```python
from build123d import *

# Parameters (mm, degrees)
SKETCH1_R           = 2.1
BOSS_EXTRUDE1_DEPTH = 2.38
BOSS_EXTRUDE2_START = 2.38
SKETCH1_3_W         = 40.25
SKETCH1_3_H         = 19.88
SKETCH1_3_W_2       = 6.925
SKETCH1_3_H_2       = 0.92
BOSS_EXTRUDE2_DEPTH = 5.72
BOSS_EXTRUDE3_START = 8.1
BOSS_EXTRUDE3_DEPTH = 2
BOSS_EXTRUDE4_START = 10.1
BOSS_EXTRUDE4_DEPTH = 0.5
BOSS_EXTRUDE5_START = 10.1
SKETCH1_6_R         = 6.5
BOSS_EXTRUDE5_DEPTH = 1.2
BOSS_EXTRUDE6_START = 10.1
SKETCH1_8_R         = 5.375
BOSS_EXTRUDE6_DEPTH = 2
BOSS_EXTRUDE7_START = 10.1
SKETCH1_9_R         = 2.95
BOSS_EXTRUDE7_DEPTH = 6.45
SKETCH1_10_W        = 40.25
SKETCH1_10_H        = 19.88
BOSS_EXTRUDE8_DEPTH = 28
CHAMFER1_SIZE       = 2
SKETCH2_W           = 6.5
SKETCH2_H           = 4
BOSS_EXTRUDE9_DEPTH = 4.75
BOSS_EXTRUDE9_TAPER = 5
CUT_EXTRUDE1_DEPTH  = 44.714035503


with BuildPart() as part:
    # Sketch1 → Boss-Extrude1 (new body)
    with BuildSketch(Plane(origin=(0, 0, 0), x_dir=(1, 0, 0), z_dir=(0, 1, 0))):
        with BuildLine():
            Line((-20.125, -9.15), (-20.125, -9.94))
            Line((-20.125, -9.94), (20.125, -9.94))
            Line((20.125, -9.94), (20.125, -9.15))
            Line((20.125, -9.15), (25.635786438, -9.15))
            ThreePointArc((25.635786438, -9.15), (26.635786438, -8.735786438), (27.05, -7.735786438))
            Line((27.05, -7.735786438), (27.05, 7.735786438))
            ThreePointArc((27.05, 7.735786438), (26.635786438, 8.735786438), (25.635786438, 9.15))
            Line((25.635786438, 9.15), (20.125, 9.15))
            Line((20.125, 9.15), (20.125, 9.94))
            Line((20.125, 9.94), (-20.125, 9.94))
            Line((-20.125, 9.94), (-20.125, 9.15))
            Line((-20.125, 9.15), (-25.635786438, 9.15))
            ThreePointArc((-25.635786438, 9.15), (-26.635786438, 8.735786438), (-27.05, 7.735786438))
            Line((-27.05, 7.735786438), (-27.05, -7.735786438))
            ThreePointArc((-27.05, -7.735786438), (-26.635786438, -8.735786438), (-25.635786438, -9.15))
            Line((-25.635786438, -9.15), (-20.125, -9.15))
        make_face()
        with BuildLine():
            ThreePointArc((-14.425, -4.627785648), (-16.045, 0), (-14.425, 4.627785648))
            Line((-14.425, 4.627785648), (-14.425, -4.627785648))
        make_face(mode=Mode.SUBTRACT)
        with Locations(Location((-24.35, -4.875, 0), (0, 0, 270))):
            Circle(SKETCH1_R, mode=Mode.SUBTRACT)
        with Locations(Location((24.35, -4.875, 0), (0, 0, 270))):
            Circle(SKETCH1_R, mode=Mode.SUBTRACT)
        with Locations(Location((-24.35, 4.875, 0), (0, 0, 270))):
            Circle(SKETCH1_R, mode=Mode.SUBTRACT)
        with Locations(Location((24.35, 4.875, 0), (0, 0, 270))):
            Circle(SKETCH1_R, mode=Mode.SUBTRACT)
    extrude(amount=BOSS_EXTRUDE1_DEPTH)

    # Sketch1<3> → Boss-Extrude2 (add)
    with BuildSketch(Plane(origin=(0, 0, 0), x_dir=(1, 0, 0), z_dir=(0, 1, 0)).offset(BOSS_EXTRUDE2_START)):
        Rectangle(SKETCH1_3_W, SKETCH1_3_H)
        with Locations((-23.5875, 0)):
            Rectangle(SKETCH1_3_W_2, SKETCH1_3_H_2)
        with Locations((23.5875, 0)):
            Rectangle(SKETCH1_3_W_2, SKETCH1_3_H_2)
    extrude(amount=BOSS_EXTRUDE2_DEPTH)

    # Sketch1<4> → Boss-Extrude3 (add)
    with BuildSketch(Plane(origin=(0, 0, 0), x_dir=(1, 0, 0), z_dir=(0, 1, 0)).offset(BOSS_EXTRUDE3_START)):
        with BuildLine():
            Line((5.758534141, 8.9), (-14.425, 8.9))
            Line((-14.425, 8.9), (-14.425, 4.627785648))
            ThreePointArc((-14.425, 4.627785648), (-16.045, 0), (-14.425, -4.627785648))
            Line((-14.425, -4.627785648), (-14.425, -8.9))
            Line((-14.425, -8.9), (5.758534141, -8.9))
            ThreePointArc((5.758534141, -8.9), (20.125, 0), (5.758534141, 8.9))
        make_face()
    extrude(amount=BOSS_EXTRUDE3_DEPTH)

    # Sketch1<5> → Boss-Extrude4 (add)
    with BuildSketch(Plane(origin=(0, 0, 0), x_dir=(1, 0, 0), z_dir=(0, 1, 0)).offset(BOSS_EXTRUDE4_START)):
        Polygon((-14.425, -8.9), (-1.425, -8.9), (-1.425, 8.9), (-14.425, 8.9), (-14.425, 4.627785648), (-14.425, -4.627785648), align=None)
    extrude(amount=BOSS_EXTRUDE4_DEPTH)

    # Sketch1<6> → Boss-Extrude5 (add)
    with BuildSketch(Plane(origin=(0, 0, 0), x_dir=(1, 0, 0), z_dir=(0, 1, 0)).offset(BOSS_EXTRUDE5_START)):
        with Locations(Location((10.185, 0, 0), (0, 0, 90))):
            Circle(SKETCH1_6_R)
    extrude(amount=BOSS_EXTRUDE5_DEPTH)

    # Sketch1<8> → Boss-Extrude6 (add)
    with BuildSketch(Plane(origin=(0, 0, 0), x_dir=(1, 0, 0), z_dir=(0, 1, 0)).offset(BOSS_EXTRUDE6_START)):
        with Locations(Location((10.185, 0, 0), (0, 0, 90))):
            Circle(SKETCH1_8_R)
    extrude(amount=BOSS_EXTRUDE6_DEPTH)

    # Sketch1<9> → Boss-Extrude7 (add)
    with BuildSketch(Plane(origin=(0, 0, 0), x_dir=(1, 0, 0), z_dir=(0, 1, 0)).offset(BOSS_EXTRUDE7_START)):
        with Locations(Location((10.185, 0, 0), (0, 0, 90))):
            Circle(SKETCH1_9_R)
    extrude(amount=BOSS_EXTRUDE7_DEPTH)

    # Sketch1<10> → Boss-Extrude8 (add)
    with BuildSketch(Plane(origin=(0, 0, 0), x_dir=(1, 0, 0), z_dir=(0, 1, 0))):
        Rectangle(SKETCH1_10_W, SKETCH1_10_H)
    extrude(amount=-BOSS_EXTRUDE8_DEPTH)

    # Chamfer1
    chamfer1_edges = [part.edges().sort_by_distance(p)[0] for p in [
        (0, -28, 9.94),
        (20.125, -28, 0),
        (-20.125, -28, 0),
        (0, -28, -9.94),
    ]]
    chamfer(chamfer1_edges, length=CHAMFER1_SIZE)

    # Sketch2 → Boss-Extrude9 (add)
    with BuildSketch(Plane(origin=(20.125, 0, 0), x_dir=(0, 0, -1), z_dir=(1, 0, 0))):
        with Locations((0, -22.1)):
            Rectangle(SKETCH2_W, SKETCH2_H)
    extrude(amount=BOSS_EXTRUDE9_DEPTH, taper=BOSS_EXTRUDE9_TAPER)

    # Sketch3 → Cut-Extrude1 (cut, through all)
    with BuildSketch(Plane(origin=(0, 0, -9.94), x_dir=(-1, 0, 0), z_dir=(0, 0, -1))):
        Polygon((-27.05, 8.1), (-27.05, 2.38), (-20.125, 3.95), (-20.125, 8.1), align=None)
        Polygon((20.125, 3.95), (27.05, 2.38), (27.05, 8.1), (20.125, 8.1), align=None)
    extrude(amount=-CUT_EXTRUDE1_DEPTH, mode=Mode.SUBTRACT)


solid = part.part
```
The listing builds one solid part. Answer for the finished solid, in the listing's coordinates (mm). A direction names the side the tool comes from. Coordinates: 2 decimals unless noted, no trailing zeros. Write each loop counter-clockwise with the first axis right and the second up, starting at its lowest first coordinate (ties: lowest second). Pieces come first, ordered by that corner, then holes.
Q1. Find the intervals of material crossed by line 1 along Z through (x, y) = (-24, 1); line 2 along Y through (x, z) = (-25, 0.5); line 3 along Y through (x, z) = (5.5, 1.5), in increasing order.
Returned:
line 1: z = -9.15 to -6.95, -2.8 to 2.8, 6.95 to 9.15
line 2: y = 0 to 2.38
line 3: y = -28 to 12.1
Q2. The mould has two halves that part along X. Classify faces 1 (the cylindrical face through (-26.65, 1.17, 8.72)), 2 (the flat face through (0, -9, -9.94)), 3 (the cylindrical face through (3.74, 10.69, 0.85)), 4 (the flat face through (24.875, -22, 0)): released by +X, released by -X, zero draft, split by the parting line, or undercut.
Returned:
face 1: released by -X
face 2: zero draft
face 3: undercut
face 4: released by +X
Q3. Section C-C, the plane y = -6.5 is taken. Write down the section's boundary in (x, z) (3 decimals).
Returned:
outline: (-20.125, -9.94) - (20.125, -9.94) - (20.125, 9.94) - (-20.125, 9.94) - close
Q4. Section D-D, the plane x = -8.5 is taken. Write down the section's boundary in (y, z), then the cut area to 3 significant figures.
Returned:
outline: (-28, -7.94) - (-26, -9.94) - (8.1, -9.94) - (8.1, -8.9) - (10.6, -8.9) - (10.6, 8.9) - (8.1, 8.9) - (8.1, 9.94) - (-26, 9.94) - (-28, 7.94) - close
area: 758 mm2
Q5. Section A-A, the plane x = 2 is taken. Write down the section's boundary in (y, z), then the cut area to 3 significant figures.
Returned:
outline: (-28, -7.94) - (-26, -9.94) - (8.1, -9.94) - (8.1, -8.9) - (10.1, -8.9) - (10.1, 8.9) - (8.1, 8.9) - (8.1, 9.94) - (-26, 9.94) - (-28, 7.94) - close
area: 749 mm2
Q6. Given P1, Ø0.8, axis at x = -23.5, y = 3, coming from the +Z side; P2, Ø2, axis at y = -12.5, z = 5, coming from the +X side (3 decimals); P3, Ø5.5, axis at x = 24.35, z = 4.875, coming from the +Y side, each flat-ended and moving along its own axis, determine where each tip first touches the part or whether it passes through.
Returned:
P1: stops at z = 0.46
P2: stops at x = 20.125
P3: stops at y = 2.38
Q7. Section B-B, the plane x = -24.35 is taken. Write down the section's boundary in (y, z) (3 decimals), then the cut area to 3 significant figures.
Returned:
outline: (0, -9.15) - (2.38, -9.15) - (2.38, -6.975) - (0, -6.975) - close; (0, -2.775) - (2.38, -2.775) - (2.38, -0.46) - (2.992, -0.46) - (2.992, 0.46) - (2.38, 0.46) - (2.38, 2.775) - (0, 2.775) - close; (0, 6.975) - (2.38, 6.975) - (2.38, 9.15) - (0, 9.15) - close
area: 24.1 mm2
Q8. Which of the six approach directions +Z, -Z, +X, -X, +Y, -Y give full straight-line access (tool end or side, diameter ignored) to faces 5 (the flat face through (-4, 9, 8.9)), 6 (the flat face through (-8, 10.6, 0)), 7 (the cylindrical face through (15.43, 11.69, 1.17)), 8 (the flat face through (18, 8.1, -8))?
Returned:
face 5: +Z, -X, +Y
face 6: +Z, -Z, -X, +Y
face 7: +Y
face 8: -Z, +X, +Y
